Verification items for the finished model (mm, model axes). A direction names the side the tool comes from. Round coordinates to 2 decimals unless told otherwise and drop trailing zeros. Return JSON: item names as keys, results as strings. Group by question number.
Item 1: Draft check along X on faces 1 (the flat face through (-155, 6, 5)), 2 (the flat face through (-50, 6, -246)), 3 (the flat face through (-2, 6, 337.5)). Enter one of: pulls with the +X half, pulls with the -X half, needs draft (parallel to the pull), parting line crosses it, or undercut.
Item 2: Access from +Z, -Z, +X, -X, +Y, -Y to the whole of each face (thin tool, end or side, straight path). Record for faces 4 (the flat face through (-2, 0, -5)), 5 (the flat face through (62, 6, 246)).
Item 3: Scan lines: probe 1 along X at (y, z) = (9, -292); probe 2 along Z at (x, y) = (-53, 2.5). Record each from-to range of solid material in increasing order. Write a range as from..to.
```python
from build123d import *

# Parameters (mm, degrees)
SKETCH1_W           = 310
SKETCH1_H           = 675
SKETCH1_W_2         = 300
SKETCH1_H_2         = 665
SKETCH1_W_3         = 260
SKETCH1_H_3         = 625
BOSS_EXTRUDE1_DEPTH = 12
SKETCH2_W           = 12
SKETCH2_H           = 12
CUT_EXTRUDE1_DEPTH  = 13
SKETCH3_W           = 12
SKETCH3_H           = 12
CUT_EXTRUDE2_DEPTH  = 13


with BuildPart() as part:
    # Sketch1 → Boss-Extrude1 (new body)
    with BuildSketch(Plane(origin=(0, 0, 0), x_dir=(1, 0, 0), z_dir=(0, 1, 0))):
        Rectangle(SKETCH1_W, SKETCH1_H)
        Rectangle(SKETCH1_W_2, SKETCH1_H_2, mode=Mode.SUBTRACT)
        Rectangle(SKETCH1_W_2, SKETCH1_H_2)
        Rectangle(SKETCH1_W_3, SKETCH1_H_3, mode=Mode.SUBTRACT)
        Rectangle(SKETCH1_W_3, SKETCH1_H_3)
    extrude(amount=BOSS_EXTRUDE1_DEPTH)

    # Sketch2 → Cut-Extrude1 (cut, through all)
    with BuildSketch(Plane(origin=(0, 12, 0), x_dir=(1, 0, 0), z_dir=(0, 1, 0))):
        with Locations((-140, -295.5)):
            Rectangle(SKETCH2_W, SKETCH2_H)
        with Locations((-140, 295.5)):
            Rectangle(SKETCH2_W, SKETCH2_H)
        with Locations((140, 295.5)):
            Rectangle(SKETCH2_W, SKETCH2_H)
        with Locations((140, -295.5)):
            Rectangle(SKETCH2_W, SKETCH2_H)
    extrude(amount=-CUT_EXTRUDE1_DEPTH, mode=Mode.SUBTRACT)

    # Sketch3 → Cut-Extrude2 (cut, through all)
    with BuildSketch(Plane(origin=(0, 12, 0), x_dir=(1, 0, 0), z_dir=(0, 1, 0))):
        with Locations((-56, -245.5)):
            Rectangle(SKETCH3_W, SKETCH3_H)
        with Locations((56, -245.5)):
            Rectangle(SKETCH3_W, SKETCH3_H)
    cut_extrude2 = extrude(amount=-CUT_EXTRUDE2_DEPTH, mode=Mode.SUBTRACT)

    # Mirror1: Cut-Extrude2 across plane
    add(cut_extrude2.mirror(Plane.XY), mode=Mode.SUBTRACT)


solid = part.part
```
Recorded:
{
 "1": {"face 1": "pulls with the -X half", "face 2": "undercut", "face 3": "needs draft"},
 "2": {"face 4": "+Z, -Z, +X, -X, -Y", "face 5": "+Y, -Y"},
 "3": {"probe 1": "-155..-146, -134..134, 146..155", "probe 2": "-337.5..-251.5, -239.5..239.5, 251.5..337.5"}
}
